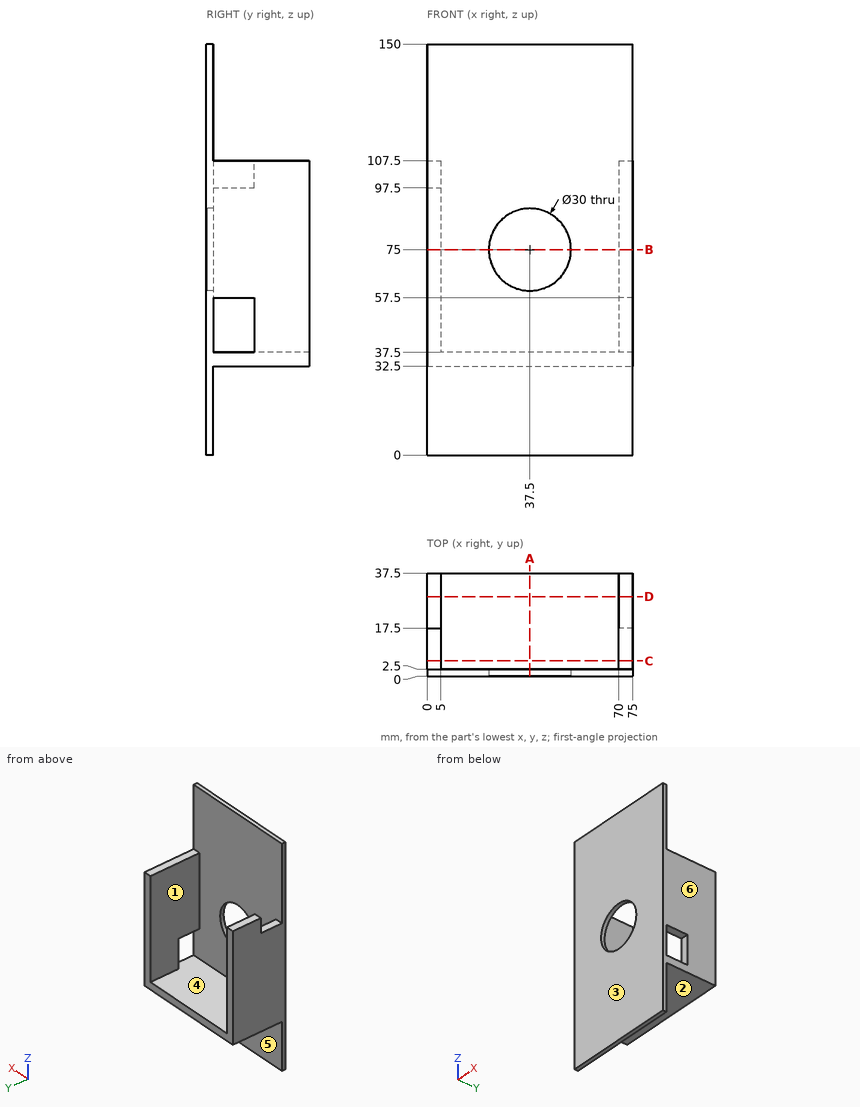
Part print with two shaded views. Sizes in mm from the minimum x, y, z corner. A direction names the side the tool comes from. Round coordinates to 2 decimals unless told otherwise and drop trailing zeros. Loops run counter-clockwise (first coordinate to the right, second up) from the corner with the lowest first, then second, coordinate; pieces in that order, holes last. Notation, with made-up numbers: (84, 3) - (118, 3) arc R35 ccw to (118, 37) - close; hole circle Ø9 at (-29, 8). An arc over 180 degrees is marked (long way). Answer as a JSON object with one key per item and string values.
Item 1: Band-saw the part on D-D on y = 29. List the corners of the cut face in (x, z), plus the area to 4 significant figures.
Output:
{"outline": "(0, 32.5) - (75, 32.5) - (75, 107.5) - (70, 107.5) - (70, 37.5) - (5, 37.5) - (5, 107.5) - (0, 107.5) - close", "area": "1,075 mm2"}
Item 2: Pin check, flat tips, straight feed: pin 1 (2 mm diameter, centred on x = 60.5, y = 24.5, fed in from +Z); pin 2 (4 mm diameter, centred on x = 2, y = 24, fed in from +Z); pin 3 (12 mm diameter, centred on x = 25.5, y = 20, fed in from -Z). Stop position of each tip, or through.
Output:
{"pin 1": "z = 37.5", "pin 2": "z = 107.5", "pin 3": "z = 32.5"}
Item 3: Pull direction X, two halves, no side cores. Call the marked faces 4, 5 and 6: pulls with the +X half, pulls with the -X half, needs draft (parallel to the pull), parting line crosses it, or undercut.
Output:
{"face 4": "undercut", "face 5": "needs draft", "face 6": "pulls with the +X half"}
Item 4: Tool access for the marked faces 1, 2 and 3: list every direction of +Z, -Z, +X, -X, +Y, -Y with a clear straight run to the whole face (end or side of a thin tool).
Output:
{"face 1": "+Z, +Y", "face 2": "-Z, +X, -X, +Y", "face 3": "+Z, -Z, +X, -X, -Y"}
Item 5: Band-saw the part on C-C on y = 5.5. List the corners of the cut face in (x, z).
Output:
{"outline": "(0, 32.5) - (75, 32.5) - (75, 37.5) - (5, 37.5) - (5, 97.5) - (0, 97.5) - close; (70, 57.5) - (75, 57.5) - (75, 107.5) - (70, 107.5) - close"}
Item 6: Wall check: L1, parallel to X at y = 4.5, z = 66; L2, parallel to Z at x = 37.5, y = 1.65; L3, parallel to Y at x = 72, z = 41. Give the ranges that are in metal, low to high.
Output:
{"L1": "0 to 5, 70 to 75", "L2": "0 to 60, 90 to 150", "L3": "0 to 2.5, 17.5 to 37.5"}
Item 7: Band-saw the part on A-A on x = 37.5. List the corners of the cut face in (y, z).
Output:
{"outline": "(0, 0) - (2.5, 0) - (2.5, 32.5) - (37.5, 32.5) - (37.5, 37.5) - (2.5, 37.5) - (2.5, 60) - (0, 60) - close; (0, 90) - (2.5, 90) - (2.5, 150) - (0, 150) - close"}
Item 8: Band-saw the part on B-B on z = 75. List the corners of the cut face in (x, y), plus the area to 4 significant figures.
Output:
{"outline": "(0, 0) - (22.5, 0) - (22.5, 2.5) - (5, 2.5) - (5, 37.5) - (0, 37.5) - close; (52.5, 0) - (75, 0) - (75, 37.5) - (70, 37.5) - (70, 2.5) - (52.5, 2.5) - close", "area": "462.5 mm2"}
